from build123d import *

# Parameters (mm, degrees)
BOSS_EXTRUDE1_DEPTH = 30
SKETCH4_R           = 1.5
CUT_EXTRUDE1_DEPTH  = 24.885599949
FILLET1_R           = 2
SKETCH5_W           = 2.5
SKETCH5_H           = 4


with BuildPart() as part:
    # Sketch3 → Boss-Extrude1 (new body)
    with BuildSketch(Plane(origin=(0, 0, 0), x_dir=(1, 0, 0), z_dir=(0, 1, 0))):
        with BuildLine():
            Line((-18.5, 38.5), (18.5, 38.5))
            Line((18.5, 38.5), (18.5, 18.5))
            Line((18.5, 18.5), (13.081475452, 13.081475452))
            ThreePointArc((13.081475452, 13.081475452), (0, 18.5), (-13.081475452, 13.081475452))
            Line((-13.081475452, 13.081475452), (-18.5, 18.5))
            Line((-18.5, 18.5), (-18.5, 38.5))
        make_face()
    extrude(amount=BOSS_EXTRUDE1_DEPTH)

    # Split1
    split(bisect_by=Plane(origin=(0, 12.373661486, -33.99635553), x_dir=(0, -0.939692621, -0.342020143), z_dir=(0, 0.342020143, -0.939692621)), keep=Keep.BOTTOM)

    # Sketch4 → Cut-Extrude1 (cut, through all)
    with BuildSketch(Plane(origin=(0, 12.373661486, -33.99635553), x_dir=(-1, 0, 0), z_dir=(0, 0.342020143, -0.939692621))):
        with Locations((9.5, 2.794891069)):
            Circle(SKETCH4_R)
        with Locations((-9.5, 2.794891069)):
            Circle(SKETCH4_R)
    extrude(amount=-CUT_EXTRUDE1_DEPTH, mode=Mode.SUBTRACT)

    # Fillet1
    fillet1_edges = [part.edges().sort_by_distance(p)[0] for p in [
        (15.790737726, 0, -15.790737726),
        (18.5, 0, -28.5),
        (-18.5, 0, -28.5),
        (-15.790737726, 0, -15.790737726),
        (0, 0, -18.5),
        (15.790737726, 30, -15.790737726),
        (18.5, 30, -23.040446486),
        (-18.5, 30, -23.040446486),
        (-15.790737726, 30, -15.790737726),
        (0, 30, -18.5),
        (13.081475452, 15, -13.081475452),
        (-13.081475452, 15, -13.081475452),
        (-18.5, 15, -18.5),
        (18.5, 15, -18.5),
        (18.5, 15, -33.040446486),
        (-18.5, 15, -33.040446486),
        (0, 30, -27.580892972),
        (0, 0, -38.5),
    ]]
    fillet(fillet1_edges, radius=FILLET1_R)

    # Sketch5 → Cut-Revolve1 (revolve, cut)
    with BuildSketch(Plane(origin=(0, 0, 0), x_dir=(0, 0, -1), z_dir=(1, 0, 0))):
        with Locations((23, 5)):
            Rectangle(SKETCH5_W, SKETCH5_H)
        with Locations((23, 25)):
            Rectangle(SKETCH5_W, SKETCH5_H)
    revolve(axis=Axis((0, 30, 0), (0, -1, 0)), mode=Mode.SUBTRACT)


solid = part.part
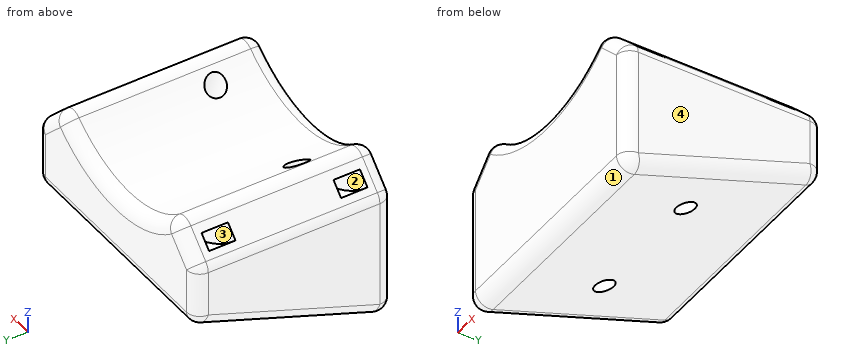
The listing builds one solid part. Answer for the finished solid, in the listing's coordinates (mm). Face numbers are marked on the shaded views. Give positions to 0.01 mm unless a question says otherwise; leave off trailing zeros. Order: outer loops, then holes, each group sorted by start corner. A loop starts at its lowest first (then second) coordinate and runs counter-clockwise, first axis right, second up. Notation, with made-up numbers: (-26.5, 40.5) - (11.5, 40.5) arc R23 ccw to (11.5, 65.5) - close; hole circle Ø1 at (3.25, -24.5). An arc over 180 degrees is marked (long way). Use one line per item in the form item = value.
1) Find section A-A on x = 0. Determine the outline of the cut face in (y, z), and give its area (3 significant figures).
Verdict:
outline = (0, -35.64) arc R2 ccw to (2.68, -37.52) - (28.68, -28.06) arc R2 ccw to (30, -26.18) - (30, -20.5) arc R2 ccw to (28, -18.5) - (2, -18.5) arc R2 ccw to (0, -20.5) - close; hole (3, -24.25) - (7, -24.25) - (7, -21.75) - (3, -21.75) - close; hole (23, -24.25) - (27, -24.25) - (27, -21.75) - (23, -21.75) - close
area = 412 mm^2
2) The mould has two halves that part along X. Classify the marked faces 1, 2, 3 and 4: released by +X, released by -X, zero draft, split by the parting line, or undercut.
Verdict:
face_1 = zero draft
face_2 = undercut
face_3 = undercut
face_4 = released by +X
3) Consider probe 1 along Y at (x, z) = (13.5, -17.5); probe 2 along Z at (x, y) = (-7, 24); probe 3 along Y at (x, z) = (-10.5, -20.5). Determine where each line is inside the solid, lowest interval first. Write a range as [from, to].
Verdict:
probe_1 = [0, 3], [7, 23], [27, 30]
probe_2 = [-29.76, -23.22], [-20.59, -17.12]
probe_3 = [0, 3], [7, 9.25], [11.63, 23], [27, 30]
4) Find section B-B on x = -10. Give the number of separate pieces and of enclosed holes in the cut face, and give its area (3 significant figures).
Verdict:
separate_pieces = 2
enclosed_holes = 2
area = 445 mm^2
5) Each of these flat-tipped pins is pushed along its axis until it touches: pin 1 (1.5 mm diameter, centred on x = -12, y = 19, fed in from +Z); pin 2 (2 mm diameter, centred on x = 9.5, y = 8, fed in from +Z); pin 3 (5 mm diameter, centred on x = 7.5, y = 6, fed in from -Z). Where does it stop, or does it pass through?
Verdict:
pin_1 = -13.86
pin_2 = -15.56
pin_3 = -37.23
